from build123d import *

# Parameters (mm, degrees)
SKETCH1_W           = 165.1
SKETCH1_H           = 114.3
BOSS_EXTRUDE1_DEPTH = 2.54
SKETCH2_W           = 17.78
SKETCH2_H           = 30.48
BOSS_EXTRUDE2_DEPTH = 27.94


with BuildPart() as part:
    # Sketch1 → Boss-Extrude1 (new body)
    with BuildSketch(Plane(origin=(0, 0, 0), x_dir=(1, 0, 0), z_dir=(0, 1, 0))):
        with Locations((16.813522013, 7.548113208)):
            Rectangle(SKETCH1_W, SKETCH1_H)
    extrude(amount=BOSS_EXTRUDE1_DEPTH)

    # Sketch2 → Boss-Extrude2 (add)
    with BuildSketch(Plane(origin=(0, 2.54, 0), x_dir=(1, 0, 0), z_dir=(0, 1, 0))):
        with Locations((65.327522013, 30.408113208)):
            Rectangle(SKETCH2_W, SKETCH2_H)
        with Locations((84.631522013, 30.408113208)):
            Rectangle(SKETCH2_W, SKETCH2_H)
        with Locations((46.023522013, 30.408113208)):
            Rectangle(SKETCH2_W, SKETCH2_H)
        with Locations((26.719522013, 30.408113208)):
            Rectangle(SKETCH2_W, SKETCH2_H)
        with Locations((7.415522013, 30.408113208)):
            Rectangle(SKETCH2_W, SKETCH2_H)
        with Locations((-11.888477987, 30.408113208)):
            Rectangle(SKETCH2_W, SKETCH2_H)
        with Locations((-31.192477987, 30.408113208)):
            Rectangle(SKETCH2_W, SKETCH2_H)
        with Locations((-50.496477987, 30.408113208)):
            Rectangle(SKETCH2_W, SKETCH2_H)
        with Locations((65.327522013, -15.311886792)):
            Rectangle(SKETCH2_W, SKETCH2_H)
        with Locations((46.023522013, -15.311886792)):
            Rectangle(SKETCH2_W, SKETCH2_H)
        with Locations((26.719522013, -15.311886792)):
            Rectangle(SKETCH2_W, SKETCH2_H)
        with Locations((7.415522013, -15.311886792)):
            Rectangle(SKETCH2_W, SKETCH2_H)
        with Locations((-11.888477987, -15.311886792)):
            Rectangle(SKETCH2_W, SKETCH2_H)
        with Locations((-31.192477987, -15.311886792)):
            Rectangle(SKETCH2_W, SKETCH2_H)
        with Locations((-50.496477987, -15.311886792)):
            Rectangle(SKETCH2_W, SKETCH2_H)
        with Locations((84.631522013, -15.311886792)):
            Rectangle(SKETCH2_W, SKETCH2_H)
    extrude(amount=BOSS_EXTRUDE2_DEPTH)


solid = part.part
Build history of the part. All positions in model axes, mm. A direction names the side the tool comes from. Give positions to 0.01 mm unless a question says otherwise; leave off trailing zeros. Order: outer loops, then holes, each group sorted by start corner. A loop starts at its lowest first (then second) coordinate and runs counter-clockwise, first axis right, second up. Notation, with made-up numbers: M 25,-4 L 47,-4 A21 ccw 47,4 Z; hole C 29,88 d1. An arc over 180 degrees is marked long. Use one line per item in the form item = value.
1) Saw through at C-C (z = 42.5). Give the cut face in (x, y), plus the area to 3 significant figures.
Calculated:
outline = M -65.74,0 L 99.36,0 L 99.36,2.54 L -65.74,2.54 Z
area = 419 mm2
2) Saw through at A-A (x = 39). Give the cut face in (y, z).
Calculated:
outline = M 0,-64.7 L 2.54,-64.7 L 2.54,-45.65 L 30.48,-45.65 L 30.48,-15.17 L 2.54,-15.17 L 2.54,0.07 L 30.48,0.07 L 30.48,30.55 L 2.54,30.55 L 2.54,49.6 L 0,49.6 Z
3) Tool access for faces 1 (the face through (-2.998, 16, -30)), 2 (the face through (65, 16, 30.552)), 3 (the face through (93.522, 16, 16)): list every direction of +Z, -Z, +X, -X, +Y, -Y with a clear straight run to the whole face (end or side of a thin tool).
Calculated:
face_1 = +Z, -Z, +Y
face_2 = +Z, +X, -X, +Y
face_3 = +Z, -Z, +X, +Y
4) Drop flat-ended pins along their axis: pin 1 (14 mm diameter, centred on x = 42.5, y = 18, fed in from -Z); pin 2 (10 mm diameter, centred on y = 20.5, z = -2.5, fed in from +X); pin 3 (9 mm diameter, centred on x = 88.5, y = 12.5, fed in from +Z). Give the stop position or say it passes through.
Calculated:
pin_1 = -45.65
pin_2 = 93.52
pin_3 = 30.55
5) Probe probe 1 along Z at (x, y) = (-33, 18.5); probe 2 along Y at (x, z) = (-1, -53.5). List the from-to ranges inside material, lowest first.
Calculated:
probe_1 = -45.65 to -15.17, 0.07 to 30.55
probe_2 = 0 to 2.54
6) Saw through at B-B (y = 15). State how many separate pieces and enclosed holes the cut face has, plus the area to 3 significant figures.
Calculated:
separate_pieces = 16
enclosed_holes = 0
area = 8,670 mm2
7) Two-plate mould, pull along Z, no slides. Class faces 4 (the face through (-51, 30.48, 15)), 5 (the face through (-51, 16, -15.168)), 6 (the face through (-12, 16, 30.552)): released by +Z, released by -Z, zero draft, split by the parting line, or undercut.
Calculated:
face_4 = zero draft
face_5 = undercut
face_6 = released by +Z
